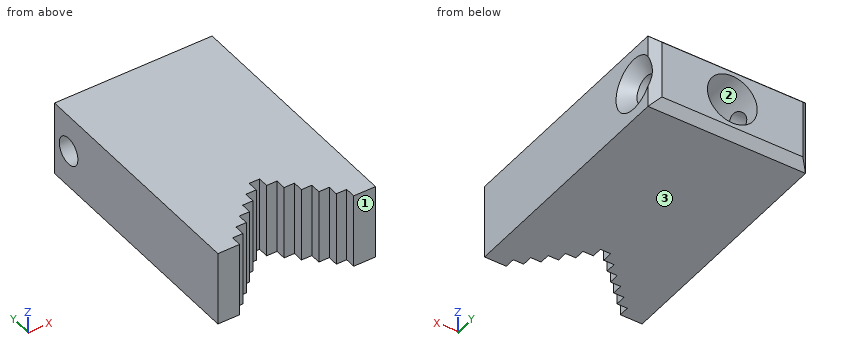
```python
from build123d import *

# Parameters (mm, degrees)
BOSS_EXTRUDE1_DEPTH                             = 9
F_12_0MM_DOWEL_HOLE1_D                          = 12
F_12_0MM_DOWEL_HOLE1_DEPTH                      = 18
F_12_0MM_DOWEL_HOLE1_TIP                        = 3.605163714
CSK_FOR_M6_FLAT_HEAD_MACHINE_SCREW2_D           = 6.6
CSK_FOR_M6_FLAT_HEAD_MACHINE_SCREW2_DEPTH       = 38
CSK_FOR_M6_FLAT_HEAD_MACHINE_SCREW2_CSINK_D     = 12.6
CSK_FOR_M6_FLAT_HEAD_MACHINE_SCREW2_CSINK_ANGLE = 90
CSK_FOR_M6_FLAT_HEAD_MACHINE_SCREW2_TIP         = 1.982840043
CHAMFER1_SIZE                                   = 2


with BuildPart() as part:
    # Sketch1 → Boss-Extrude1 (new, symmetric)
    with BuildSketch(Plane.XY):
        Polygon((19, 60), (-19, 60), (-19, 0), (-13.75, 0), (-13.75, 2.5), (-11.25, 2.5), (-11.25, 5), (-8.75, 5), (-8.75, 7.5), (-6.25, 7.5), (-6.25, 10), (-3.75, 10), (-3.75, 12.5), (-1.25, 12.5), (-1.25, 15), (1.25, 15), (1.25, 12.5), (3.75, 12.5), (3.75, 10), (6.25, 10), (6.25, 7.5), (8.75, 7.5), (8.75, 5), (11.25, 5), (11.25, 2.5), (13.75, 2.5), (13.75, 0), (19, 0), align=None)
    extrude(amount=BOSS_EXTRUDE1_DEPTH, both=True)

    # Ø12.0mm Dowel Hole1
    with Locations(Plane(origin=(0, 60, 0), x_dir=(1, 0, 0), z_dir=(0, 1, 0))):
        with Locations((0, 0)):
            Hole(F_12_0MM_DOWEL_HOLE1_D / 2, depth=F_12_0MM_DOWEL_HOLE1_DEPTH)
            with Locations((0, 0, -(F_12_0MM_DOWEL_HOLE1_DEPTH + F_12_0MM_DOWEL_HOLE1_TIP / 2))):  # 118° drill point
                Cone(0, F_12_0MM_DOWEL_HOLE1_D / 2, F_12_0MM_DOWEL_HOLE1_TIP, mode=Mode.SUBTRACT)

    # CSK for M6 Flat Head Machine Screw2
    with Locations(Plane(origin=(19, 0, 0), x_dir=(0, 0, -1), z_dir=(1, 0, 0))):
        with Locations((0, 53)):
            CounterSinkHole(CSK_FOR_M6_FLAT_HEAD_MACHINE_SCREW2_D / 2, CSK_FOR_M6_FLAT_HEAD_MACHINE_SCREW2_CSINK_D / 2, depth=CSK_FOR_M6_FLAT_HEAD_MACHINE_SCREW2_DEPTH, counter_sink_angle=CSK_FOR_M6_FLAT_HEAD_MACHINE_SCREW2_CSINK_ANGLE)
            with Locations((0, 0, -(CSK_FOR_M6_FLAT_HEAD_MACHINE_SCREW2_DEPTH + CSK_FOR_M6_FLAT_HEAD_MACHINE_SCREW2_TIP / 2))):  # 118° drill point
                Cone(0, CSK_FOR_M6_FLAT_HEAD_MACHINE_SCREW2_D / 2, CSK_FOR_M6_FLAT_HEAD_MACHINE_SCREW2_TIP, mode=Mode.SUBTRACT)

    # Chamfer1
    # the kernel refuses this chamfer: 2 mm, written as the material it takes off along each edge
    with BuildSketch(Plane(origin=(24.143365976, 60, -9), x_dir=(0, 0.027495876610585623, 0.9996219169112968), z_dir=(-1, 0, 0))) as chamfer1_piece_1:
        Polygon((CHAMFER1_SIZE * 0.999621916911, -CHAMFER1_SIZE * 0.0274958766106), (-CHAMFER1_SIZE * 0.0274958766106, -CHAMFER1_SIZE * 0.999621916911), (0, 0), align=None)
    extrude(amount=48.286731952, mode=Mode.SUBTRACT)
    with BuildSketch(Plane(origin=(-19, 60, -14.143365976), x_dir=(-0.027495876610585647, -0.9996219169112968, 0), z_dir=(0, 0, 1)), Plane(origin=(19, 60, -14.143365976), x_dir=(-0.9996219169112968, 0.027495876610585647, 0), z_dir=(0, 0, 1))) as chamfer1_piece_2:
        Polygon((CHAMFER1_SIZE * 0.999621916911, CHAMFER1_SIZE * 0.0274958766106), (-CHAMFER1_SIZE * 0.0274958766106, CHAMFER1_SIZE * 0.999621916911), (0, 0), align=None)
    extrude(amount=28.286731952, mode=Mode.SUBTRACT)
    with BuildSketch(Plane(origin=(24.143365976, 60, 9), x_dir=(0, 0.027495876610585623, -0.9996219169112968), z_dir=(-1, 0, 0))) as chamfer1_piece_3:
        Polygon((CHAMFER1_SIZE * 0.999621916911, CHAMFER1_SIZE * 0.0274958766106), (-CHAMFER1_SIZE * 0.0274958766106, CHAMFER1_SIZE * 0.999621916911), (0, 0), align=None)
    extrude(amount=48.286731952, mode=Mode.SUBTRACT)


solid = part.part
```
CAD build for the part. Positions are in the model's coordinates, mm. Face numbers are marked on the shaded views. Round coordinates to 2 decimals unless told otherwise and drop trailing zeros. Order: outer loops, then holes, each group sorted by start corner. A loop starts at its lowest first (then second) coordinate and runs counter-clockwise, first axis right, second up. Notation, with made-up numbers: (77.25, 69.5) - (116.25, 69.5) arc R20 ccw to (116.25, 85.5) - close; hole circle Ø4 at (35, -29). An arc over 180 degrees is marked (long way). Answer in a Markdown table with one row per item. Add a question column.
(1) Mould opens along Z. For the marked faces 1, 2 and 3 say: +Z half, -Z half, draft (parallel to the pull), parting line (faces both ways), or undercut.
(2) Band-saw the part on D-D on x = 15. List the corners of the cut face in (y, z).
(3) Band-saw the part on B-B on x = -13. List the corners of the cut face in (y, z).
(4) Drop flat-ended pins along their axis: pin 1 Ø1.2 at (x, z) = (-0.5, 2) entering from -Y; pin 2 Ø1.2 at (x, z) = (-4.5, -1.5) entering from -Y; pin 3 Ø7.5 at (y, z) = (53, 0) entering from +X. Give the stop position or say it passes through.
(5) Band-saw the part on C-C on z = 0.75. Count the separate pieces of the cut face and the enclosed holes in it, and give its area (3 significant figures).
(6) Band-saw the part on A-A on y = 53. List the corners of the cut face in (x, z), and give its area (3 significant figures).
(7) Probe L1, parallel to Z at x = 8, y = 53; L2, parallel to Y at x = 7.5, z = 0; L3, parallel to X at y = 6.5, z = 3.75. List the from-to ranges inside material, lowest first. Write a range as [from, to].
Data:
| question | item | result |
|---|---|---|
| 1 | face 1 | draft |
| 1 | face 2 | undercut |
| 1 | face 3 | -Z half |
| 2 | outline | (0, -9) - (58, -9) - (60, -7) - (60, 7) - (58, 9) - (0, 9) - close; hole circle Ø6.6 at (53, 0) |
| 3 | outline | (2.5, -9) - (58, -9) - (60, -7) - (60, 7) - (58, 9) - (2.5, 9) - close; hole circle Ø6.6 at (53, 0) |
| 4 | pin 1 | stops at y = 15 |
| 4 | pin 2 | stops at y = 10 |
| 4 | pin 3 | stops at x = 16.45 |
| 5 | separate pieces | 3 |
| 5 | enclosed holes | 0 |
| 5 | area | 1,640 mm^2 |
| 6 | outline | (-19, -9) - (19, -9) - (19, -6.3) - (16, -3.3) - (5.01, -3.3) arc R6 cw to (-5.01, -3.3) - (-19, -3.3) - close; (-19, 3.3) - (-5.01, 3.3) arc R6 cw to (5.01, 3.3) - (16, 3.3) - (19, 6.3) - (19, 9) - (-19, 9) - close |
| 6 | area | 386 mm^2 |
| 7 | L1 | z = [-9, -3.3], [3.3, 9] |
| 7 | L2 | y = [7.5, 49.7], [56.3, 60] |
| 7 | L3 | x = [-19, -8.75], [8.75, 19] |
